Could you check a few things on this model? Use its own coordinates, in mm. A direction names the side the tool comes from. Coordinates: 2 decimals unless noted, no trailing zeros. Loops run counter-clockwise (first coordinate to the right, second up) from the corner with the lowest first, then second, coordinate; pieces in that order, holes last. Notation, with made-up numbers: (-8.75, 30) -> (-1.75, 30) arc R11 ccw to (-1.75, 50) -> close; hole circle Ø10 at (7, -39.5). An arc over 180 degrees is marked (long way). One line per question, with ' | ' between items.
```python
from build123d import *

# Parameters (mm, degrees)
F1_DEPTH = 15.85
F2_R     = 1.9679985055
F2_R_2   = 1.968
F3_DEPTH = 2
F5_DEPTH = 5


with BuildPart() as f1:
    # F0 (on Right) → F1 (new body)
    with BuildSketch(Plane.YZ):
        Polygon((-17.2513356102, 38.1256241769), (-17.2513356102, 47.7256241769), (-25.6513356102, 47.7256241769), (-32.7313356102, 39.7056241769), (-32.7313356102, 38.1256241769), align=None)
    extrude(amount=F1_DEPTH)

    # F2 (on face) → F3 (join)
    with BuildSketch(Plane.XY.offset(47.7256241769)):
        with Locations((3.9679985055, -21.0531856865)):
            Circle(F2_R)
        with Locations((11.882, -20.9530331194)):
            Circle(F2_R_2)
    extrude(amount=F3_DEPTH)

    # F4 (on face) → F5 (cut)
    with BuildSketch(Plane(origin=(0, 0, 38.1256241769), x_dir=(1, 0, 0), z_dir=(0, 0, -1))):
        with BuildLine():
            Line((7.0497745559, 25.9519131103), (1, 32.0581247445))
            Line((1, 32.0581247445), (1, 18.0789209985))
            Line((1, 18.0789209985), (7.0497745559, 24.1851326327))
            ThreePointArc((7.0497745559, 24.1851326327), (6.6814575231, 25.0685228715), (7.0497745559, 25.9519131103))
        make_face()
        with BuildLine():
            Line((14.85, 32.0581247445), (1, 32.0581247445))
            Line((1, 32.0581247445), (7.0497745559, 25.9519131103))
            ThreePointArc((7.0497745559, 25.9519131103), (7.925, 26.3120653484), (8.8002254441, 25.9519131103))
            Line((8.8002254441, 25.9519131103), (14.85, 32.0581247445))
        make_face()
        with BuildLine():
            Line((14.85, 21.5539868837), (14.85, 32.0581247445))
            Line((14.85, 32.0581247445), (8.8002254441, 25.9519131103))
            ThreePointArc((8.8002254441, 25.9519131103), (9.072775655, 25.5470716544), (9.1685424769, 25.0685228715))
            ThreePointArc((9.1685424769, 25.0685228715), (9.072775655, 24.5899740886), (8.8002254441, 24.1851326327))
            Line((8.8002254441, 24.1851326327), (14.85, 18.0789209985))
            Line((14.85, 18.0789209985), (14.85, 21.5539868837))
        make_face()
        with BuildLine():
            Line((7.0497745559, 24.1851326327), (1, 18.0789209985))
            Line((1, 18.0789209985), (14.85, 18.0789209985))
            Line((14.85, 18.0789209985), (8.8002254441, 24.1851326327))
            ThreePointArc((8.8002254441, 24.1851326327), (7.925, 23.8249803946), (7.0497745559, 24.1851326327))
        make_face()
        with BuildLine():
            Line((7.925, 25.0685228715), (7.2684074253, 24.4058050824))
            ThreePointArc((7.2684074253, 24.4058050824), (7.925, 24.1356195125), (8.5815925747, 24.4058050824))
            Line((8.5815925747, 24.4058050824), (7.925, 25.0685228715))
        make_face()
        with BuildLine():
            Line((7.925, 25.0685228715), (7.2684074253, 25.7312406607))
            ThreePointArc((7.2684074253, 25.7312406607), (6.992096641, 25.0685228715), (7.2684074253, 24.4058050824))
            Line((7.2684074253, 24.4058050824), (7.925, 25.0685228715))
        make_face()
        with BuildLine():
            ThreePointArc((8.5815925747, 25.7312406607), (7.925, 26.0014262305), (7.2684074253, 25.7312406607))
            Line((7.2684074253, 25.7312406607), (7.925, 25.0685228715))
            Line((7.925, 25.0685228715), (8.5815925747, 25.7312406607))
        make_face()
        with BuildLine():
            ThreePointArc((8.857903359, 25.0685228715), (8.7860592592, 25.4275293191), (8.5815925747, 25.7312406607))
            Line((8.5815925747, 25.7312406607), (7.925, 25.0685228715))
            Line((7.925, 25.0685228715), (8.5815925747, 24.4058050824))
            ThreePointArc((8.5815925747, 24.4058050824), (8.7860592592, 24.7095164239), (8.857903359, 25.0685228715))
        make_face()
    extrude(amount=-F5_DEPTH, mode=Mode.SUBTRACT)


solid = f1.part
```
Q1. For faces 4 (the face through (8, -32.058, 39)), 5 (the face through (3.541, -22.974, 48.712)), 6 (the face through (8, -25, 43.126)), which set-ups out of +Z, -Z, +X, -X, +Y, -Y let a thin tool reach every point of the face, with its end or its side?
Values follow:
face 4: +Z, -Z | face 5: +Z | face 6: -Z
Q2. Imagine slicing it at B-B on z = 42.5. Write out the boundary of the cut face in (x, y) (3 decimals).
Values follow:
outline: (0, -30.264) -> (1, -30.264) -> (1, -18.079) -> (14.85, -18.079) -> (14.85, -30.264) -> (15.85, -30.264) -> (15.85, -17.251) -> (0, -17.251) -> close; circle Ø2.487 at (7.925, -25.069); hole circle Ø1.866 at (7.925, -25.069)
Q3. Please list where these lines run through material, in increasing order: L1, parallel to X at y = -23, z = 43; L2, parallel to Y at x = 10, z = 39.25; L3, parallel to X at y = -25.75, z = 40.25. Write a range as [from, to].
Values follow:
L1: x = [0, 1], [14.85, 15.85] | L2: y = [-32.73, -32.06], [-18.08, -17.25] | L3: x = [0, 1], [6.88, 7.29], [8.56, 8.97], [14.85, 15.85]
Q4. Imagine slicing it at C-C on x = 4.25. Write out the boundary of the cut face in (y, z), plus the area to 3 significant figures.
Values follow:
outline: (-32.73, 38.13) -> (-32.06, 38.13) -> (-32.06, 40.47) -> (-32.73, 39.71) -> close; (-29.71, 43.13) -> (-18.08, 43.13) -> (-18.08, 38.13) -> (-17.25, 38.13) -> (-17.25, 47.73) -> (-19.11, 47.73) -> (-19.11, 49.73) -> (-23, 49.73) -> (-23, 47.73) -> (-25.65, 47.73) -> close | area: 61.2 mm2
Q5. For pin 1 (6 mm diameter, centred on x = 12, y = -28, fed in from +Z); pin 2 (3 mm diameter, centred on x = 9.5, z = 45.5, fed in from -Y); pin 3 (6 mm diameter, centred on x = 9, y = -21.5, fed in from -Z); pin 4 (0.9 mm diameter, centred on x = 8, y = -25, fed in from -Z), each with a flat end and sliding along its axis, tell me the tip position at first contact or that it passes through.
Values follow:
pin 1: stops at z = 47.73 | pin 2: stops at y = -28.94 | pin 3: stops at z = 38.13 | pin 4: stops at z = 43.13
Q6. We'd pull the mould along X, two halves only. Please class faces 1 (the face through (0, -23, 43)), 2 (the face through (15.85, -23, 43)), 3 (the face through (14.85, -25, 41)): released by +X, released by -X, zero draft, split by the parting line, or undercut.
Values follow:
face 1: released by -X | face 2: released by +X | face 3: undercut
Q7. Imagine slicing it at D-D on y = -28.75. Write out the boundary of the cut face in (x, z), plus the area to 3 significant figures.
Values follow:
outline: (0, 38.13) -> (1, 38.13) -> (1, 43.13) -> (14.85, 43.13) -> (14.85, 38.13) -> (15.85, 38.13) -> (15.85, 44.22) -> (0, 44.22) -> close | area: 27.3 mm2
Q8. Imagine slicing it at A-A on z = 39. Write out the boundary of the cut face in (x, y) (3 decimals), plus the area to 3 significant figures.
Values follow:
outline: (0, -32.731) -> (15.85, -32.731) -> (15.85, -17.251) -> (0, -17.251) -> close; circle Ø2.487 at (7.925, -25.069); hole (1, -32.058) -> (14.85, -32.058) -> (14.85, -18.079) -> (1, -18.079) -> close; hole circle Ø1.866 at (7.925, -25.069) | area: 53.9 mm2
